```python
from build123d import *

# Parameters (mm, degrees)
SKETCH_1_W          = 23.757047591
SKETCH_1_H          = 23.75704759
EXTRUDE_1_DEPTH     = 3
SKETCH_2_W          = 2.229782935
SKETCH_2_H          = 144.701322111
EXTRUDE_2_DEPTH     = 115
FILLET_1_R          = 20
SKETCH_3_W          = 17.433740909
SKETCH_3_H          = 91.487428691
CUT_EXTRUDE_1_DEPTH = 75
FILLET_2_R          = 10
FILLET_3_R          = 10


with BuildPart() as part:
    # 草图1 → 凸台-拉伸1 (new body)
    with BuildSketch(Plane.XY):
        with Locations((-21.874536556, 0.392800792)):
            Rectangle(SKETCH_1_W, SKETCH_1_H)
    extrude(amount=EXTRUDE_1_DEPTH)

    # 草图2 → 凸台-拉伸2 (add)
    with BuildSketch(Plane.XY.offset(3)):
        with Locations((-22.937382742, -43.600525925)):
            Rectangle(SKETCH_2_W, SKETCH_2_H)
    extrude(amount=EXTRUDE_2_DEPTH)

    # 圆角1
    # the kernel refuses this fillet: 20 mm, written as the material it adds along each edge
    with BuildSketch(Plane(origin=(-24.052274209, -11.485723003, 3), x_dir=(-1, 0, 0), z_dir=(0, 1, 0))) as fillet_1_piece_1:
        with BuildLine():
            CenterArc((20, 17.144275835), FILLET_1_R, 180, 59.005172318)
            Line((0, 17.144275835), (0, 0))
            Line((0, 0), (9.700786142, 0))
        make_face()
    extrude(amount=23.75704759)

    # 草图3 → 切除-拉伸1 (cut)
    with BuildSketch(Plane(origin=(-21.822491274, 0, 0), x_dir=(0, 0, -1), z_dir=(1, 0, 0))):
        with Locations((-8.716870455, -71.123991133)):
            Rectangle(SKETCH_3_W, SKETCH_3_H)
    extrude(amount=-CUT_EXTRUDE_1_DEPTH, mode=Mode.SUBTRACT)

    # 圆角2
    fillet_2_edges = [part.edges().sort_by_distance(p)[0] for p in [
        (-22.937382741, -25.380276788, 17.433740909),
    ]]
    fillet(fillet_2_edges, radius=FILLET_2_R)

    # 圆角3
    fillet_3_edges = [part.edges().sort_by_distance(p)[0] for p in [
        (-22.937382741, -25.380276788, 3),
    ]]
    fillet(fillet_3_edges, radius=FILLET_3_R)


solid = part.part
```
Design review of the part built by this model. Coordinates are the model's own, in mm. A direction names the side the tool comes from. Give positions to 0.01 mm unless a question says otherwise; leave off trailing zeros. Write each loop counter-clockwise with the first axis right and the second up, starting at its lowest first coordinate (ties: lowest second). Pieces come first, ordered by that corner, then holes. Notation, with made-up numbers: (15.25, 28) -> (63.25, 28) arc R29 ccw to (63.25, 60) -> close; hole circle Ø3 at (-5, -21). An arc over 180 degrees is marked (long way). Answer in a Markdown table with one row per item.
(1) Consider section B-B (x = -19.25). State the section outline as (y, z) points.
Results:
| item | result |
|---|---|
| outline | (-11.49, 0) -> (12.27, 0) -> (12.27, 3) -> (-11.49, 3) -> close |
(2) Clearance check with flat-ended pins moving along their axes: pin 1 (3 mm diameter, centred on y = -54, z = 66, fed in from -X); pin 2 (12 mm diameter, centred on y = -69.5, z = 58.5, fed in from +X); pin 3 (0.7 mm diameter, centred on x = -22.5, y = -13, fed in from -Z); pin 4 (10 mm diameter, centred on x = -30, y = -69, fed in from -Z). State where each tip first meets the part, or that it passes through.
Results:
| item | result |
|---|---|
| pin 1 | x = -24.05 |
| pin 2 | x = -21.82 |
| pin 3 | z = 3 |
| pin 4 | through |
(3) For faces 1 (the flat face through (-16, 1, 3)), 2 (the cylindrical face through (-26.575, 0.227, 10.421)), list the 3-axis set-ups (+Z, -Z, +X, -X, +Y, -Y) from which the entire face can be reached by the end or side of a thin tool; tool diameter is ignored.
Results:
| item | result |
|---|---|
| face 1 | +Z, +X, +Y, -Y |
| face 2 | +Z, -X, +Y, -Y |
(4) Consider section C-C (z = 89.5). State the section outline as (x, y) points, then the cut area to 3 significant figures.
Results:
| item | result |
|---|---|
| outline | (-24.05, -115.95) -> (-21.82, -115.95) -> (-21.82, 28.75) -> (-24.05, 28.75) -> close |
| area | 323 mm2 |
(5) Consider section A-A (y = 4). State the section outline as (x, z) points.
Results:
| item | result |
|---|---|
| outline | (-33.75, 0) -> (-10, 0) -> (-10, 3) -> (-21.82, 3) -> (-21.82, 118) -> (-24.05, 118) -> (-24.05, 20.14) arc R20 cw to (-33.75, 3) -> close |
(6) To check wall thickness, follow probe 1 along X at (y, z) = (-13.5, 7.5); probe 2 along Z at (x, y) = (-22.5, -71). State the ranges of each line that lie inside material, in increasing order.
Results:
| item | result |
|---|---|
| probe 1 | -24.05 to -21.82 |
| probe 2 | 17.43 to 118 |
